Build history of the part. All positions in model axes, mm. Face numbers are marked on the shaded views. A direction names the side the tool comes from. Give positions to 0.01 mm unless a question says otherwise; leave off trailing zeros. Loops run counter-clockwise (first coordinate to the right, second up) from the corner with the lowest first, then second, coordinate; pieces in that order, holes last. Notation, with made-up numbers: M 3.5,1.5 L 50.5,1.5 A25 cw 50.5,32.5 Z; hole C -8.5,9 d5. An arc over 180 degrees is marked long. Answer as a JSON object with one key per item and string values. Group by question number.
1. 3-axis set-ups, long thin cutter, end or side, ignore diameter. For the marked faces 1, 2 and 3: which of +Z, -Z, +X, -X, +Y, -Y reach the whole face in a straight line?
2. Slice it at B-B (y = 11). List the corners of the cut face in (x, z), then the cut area to 3 significant figures.
3. Drill centre lines: line 1 along Y through (x, z) = (-1.05, 1.85); line 2 along X through (y, z) = (0.5, 1.85); line 3 along X through (y, z) = (11.25, -1.7). Where is each one in solid material? Low to high. Write a range as [from, to].
4. Slice it at A-A (x = 0). List the corners of the cut face in (y, z), then the cut area to 3 significant figures.
5. Slice it at C-C (z = 2.1). List the corners of the cut face in (x, y), then the cut area to 3 significant figures.
6. Slice it at D-D (x = -1.2). List the corners of the cut face in (y, z).
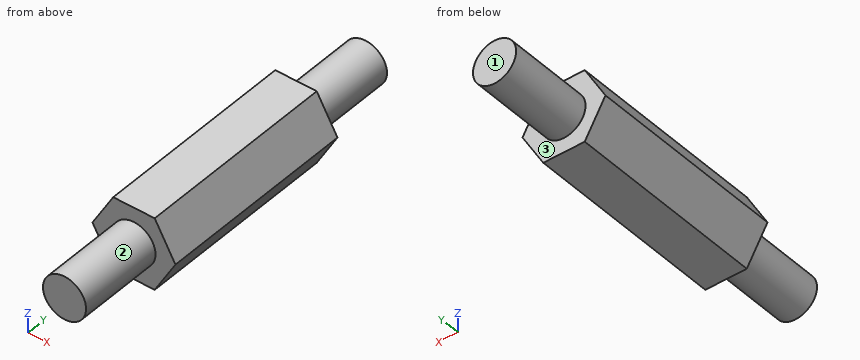
Autodesk Inventor part; units mm, degrees
ref_plane "YZ Plane" through (0, 0, 0) normal (1, 0, 0) x (0, 1, 0)
ref_plane "XZ Plane" through (0, 0, 0) normal (0, 1, 0) x (-1, 0, 0)
ref_plane "XY Plane" through (0, 0, 0) normal (0, 0, 1) x (1, 0, 0)
sketch "草圖2" plane through (0, 0, 0) normal (0, 1, 0) x (-1, 0, 0)
  line L0 (-2.8868, 0) -> (-1.4434, 2.5)
  line L1 (-1.4434, 2.5) -> (1.4434, 2.5)
  line L2 (1.4434, 2.5) -> (2.8868, 0)
  line L3 (2.8868, 0) -> (1.4434, -2.5)
  line L4 (1.4434, -2.5) -> (-1.4434, -2.5)
  line L5 (-1.4434, -2.5) -> (-2.8868, 0)
  point P0 (0, 0)
  point P1 (0, 0)
  dimension "d2" = 5
extrude "擠出1" add sketch "草圖2" along normal blind 14
sketch "草圖3" plane through (0, 0, 0) normal (0, 0, 1) x (1, 0, 0)
  line L0 (1.4434, 14) -> (-1.4434, 14)
  line L1 (0, 14) -> (1.5, 14)
  line L2 (1.5, 14) -> (1.5, 20)
  line L3 (1.5, 20) -> (0, 20)
  line L4 (0, 20) -> (0, 14)
  line L5 (0, 17.268) -> (0, -3.3114)
  line L6 (0, 0) -> (1.5, 0)
  line L7 (1.5, 0) -> (1.5, -6)
  line L8 (1.5, -6) -> (0, -6)
  line L9 (0, -6) -> (0, 0)
  point P0 (0.75, 20)
  dimension "d5" = 3
  dimension "d6" = 6
  dimension "d8" = 6
revolve "迴轉1" add sketch "草圖3" angle 360 about axis through (0, 17.268, 0) along (0, -1, 0)
properties part number "copper_pillar_M3_L15" material "Copper"
Established:
{
 "1": {"face 1": "+Z, -Z, +X, -X, +Y", "face 2": "-Y", "face 3": "+Y"},
 "2": {"outline": "M -2.89,0 L -1.44,-2.5 L 1.44,-2.5 L 2.89,0 L 1.44,2.5 L -1.44,2.5 Z", "area": "21.7 mm^2"},
 "3": {"line 1": "y = [0, 14]", "line 2": "x = [-1.82, 1.82]", "line 3": "x = [-1.91, 1.91]"},
 "4": {"outline": "M -6,-1.5 L 0,-1.5 L 0,-2.5 L 14,-2.5 L 14,-1.5 L 20,-1.5 L 20,1.5 L 14,1.5 L 14,2.5 L 0,2.5 L 0,1.5 L -6,1.5 Z", "area": "106 mm^2"},
 "5": {"outline": "M -1.67,0 L 1.67,0 L 1.67,14 L -1.67,14 Z", "area": "46.9 mm^2"},
 "6": {"outline": "M -6,-0.9 L 0,-0.9 L 0,-2.5 L 14,-2.5 L 14,-0.9 L 20,-0.9 L 20,0.9 L 14,0.9 L 14,2.5 L 0,2.5 L 0,0.9 L -6,0.9 Z"}
}
